Input: part model. Units: mm. Frame: model coordinates. A direction names the side the tool comes from. Coordinates: 2 decimals unless noted, no trailing zeros. Loops run counter-clockwise (first coordinate to the right, second up) from the corner with the lowest first, then second, coordinate; pieces in that order, holes last.
(1) Set-up query: faces 1 (the face through (-9, -5, 3)), 2 (the face through (5, -8, 3)), 3 (the face through (0, 5, 3)). Return all of +Z, -Z, +X, -X, +Y, -Y with unobstructed straight access to the full face (end or side cutting, diameter ignored); none if empty.
(2) Line query: L1, parallel to Y at x = -9.25, z = 3.1; L2, parallel to X at y = 2.5, z = 5.55. Output: solid intervals per line, ascending.
(3) Section B-B, the plane x = -8. Return loops of the section in (y, z).
(4) Contact query for flat-ended pins moving along their axis: P1, Ø2, axis at y = -7, z = 3.5, coming from the -X side; P2, Ø3, axis at y = -8, z = 2.5, coming from the +X side; P3, Ø1.8, axis at x = -7, z = 2, coming from the -Y side. Output: stop coordinate, or through.
(5) Section A-A, the plane z = 2.4. Return loops of the section in (x, y), then the cut area to 3 significant figures.
```python
from build123d import *

# Parameters (mm, degrees)
BOSS_EXTRU_1_DEPTH = 6
CONG_1_R           = 3


with BuildPart() as part:
    # Esquisse1 → Boss.-Extru.1 (new body)
    with BuildSketch(Plane.XY):
        Polygon((5, -5), (12.5, -5), (12.5, 5), (-12.5, 5), (-12.5, -5), (-5, -5), (-5, -11), (5, -11), align=None)
    extrude(amount=BOSS_EXTRU_1_DEPTH)

    # Congé1
    cong_1_edges = [part.edges().sort_by_distance(p)[0] for p in [
        (-12.5, 5, 3),
        (12.5, 5, 3),
    ]]
    fillet(cong_1_edges, radius=CONG_1_R)


solid = part.part
```
Report:
1. face 1: +Z, -Z, -X, -Y
1. face 2: +Z, -Z, +X, -Y
1. face 3: +Z, -Z, +X, -X, +Y
2. L1: y = -5 to 5
2. L2: x = -12.46 to 12.46
3. outline: (-5, 0) - (5, 0) - (5, 6) - (-5, 6) - close
4. P1: stops at x = -5
4. P2: stops at x = 5
4. P3: stops at y = -5
5. outline: (-12.5, -5) - (-5, -5) - (-5, -11) - (5, -11) - (5, -5) - (12.5, -5) - (12.5, 2) arc R3 ccw to (9.5, 5) - (-9.5, 5) arc R3 ccw to (-12.5, 2) - close
5. area: 306 mm2
